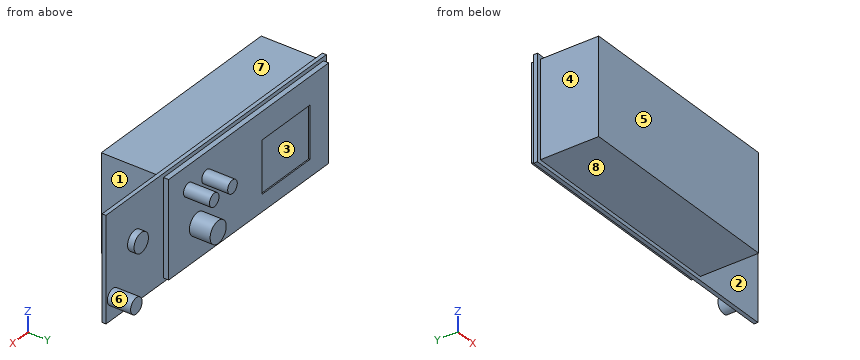
```python
from build123d import *

# Parameters (mm, degrees)
SKETCH_1_W          = 230
SKETCH_1_H          = 80
EXTRUDE_1_DEPTH     = 3
SKETCH_2_W          = 167
SKETCH_2_H          = 74
EXTRUDE_2_DEPTH     = 4
SKETCH_3_W          = 50
SKETCH_3_H          = 40
CUT_EXTRUDE_1_DEPTH = 1
SKETCH_4_R          = 8.4
EXTRUDE_3_DEPTH     = 16
SKETCH_5_R          = 5
EXTRUDE_4_DEPTH     = 20
SKETCH_6_R          = 6
EXTRUDE_5_DEPTH     = 18
SKETCH_7_R          = 7.5
EXTRUDE_6_DEPTH     = 5
SKETCH_8_W          = 167
SKETCH_8_H          = 74
EXTRUDE_7_DEPTH     = 45


with BuildPart() as part:
    # 草图1 → 凸台-拉伸1 (new body)
    with BuildSketch(Plane(origin=(0, 0, 0), x_dir=(1, 0, 0), z_dir=(0, 1, 0))):
        with Locations((35.37586548, -1.78041543)):
            Rectangle(SKETCH_1_W, SKETCH_1_H)
    extrude(amount=EXTRUDE_1_DEPTH)

    # 草图2 → 凸台-拉伸2 (add)
    with BuildSketch(Plane(origin=(0, 3, 0), x_dir=(1, 0, 0), z_dir=(0, 1, 0))):
        with Locations((6.87586548, -1.78041543)):
            Rectangle(SKETCH_2_W, SKETCH_2_H)
    extrude(amount=EXTRUDE_2_DEPTH)

    # 草图3 → 切除-拉伸1 (cut)
    with BuildSketch(Plane(origin=(0, 7, 0), x_dir=(1, 0, 0), z_dir=(0, 1, 0))):
        with Locations((-32.02413452, 2.21958457)):
            Rectangle(SKETCH_3_W, SKETCH_3_H)
    extrude(amount=-CUT_EXTRUDE_1_DEPTH, mode=Mode.SUBTRACT)

    # 草图4 → 凸台-拉伸3 (add)
    with BuildSketch(Plane(origin=(0, 7, 0), x_dir=(1, 0, 0), z_dir=(0, 1, 0))):
        with Locations(Location((60.37586548, 9.21958457, 0), (0, 0, 270))):
            Circle(SKETCH_4_R)
    extrude(amount=EXTRUDE_3_DEPTH)

    # 草图5 → 凸台-拉伸4 (add)
    with BuildSketch(Plane(origin=(0, 7, 0), x_dir=(1, 0, 0), z_dir=(0, 1, 0))):
        with Locations(Location((50.87586548, -20.78041543, 0), (0, 0, 270))):
            Circle(SKETCH_5_R)
        with Locations(Location((69.87586548, -20.78041543, 0), (0, 0, 270))):
            Circle(SKETCH_5_R)
    extrude(amount=EXTRUDE_4_DEPTH)

    # 草图6 → 凸台-拉伸5 (add)
    with BuildSketch(Plane(origin=(0, 3, 0), x_dir=(1, 0, 0), z_dir=(0, 1, 0))):
        with Locations(Location((143.07586548, 21.71958457, 0), (0, 0, 270))):
            Circle(SKETCH_6_R)
    extrude(amount=EXTRUDE_5_DEPTH)

    # 草图7 → 凸台-拉伸6 (add)
    with BuildSketch(Plane(origin=(0, 3, 0), x_dir=(1, 0, 0), z_dir=(0, 1, 0))):
        with Locations(Location((120.37586548, -8.108420441, 0), (0, 0, 270))):
            Circle(SKETCH_7_R)
    extrude(amount=EXTRUDE_6_DEPTH)

    # 草图8 → 凸台-拉伸7 (add)
    with BuildSketch(Plane.XZ):
        with Locations((6.87586548, 1.78041543)):
            Rectangle(SKETCH_8_W, SKETCH_8_H)
    extrude(amount=EXTRUDE_7_DEPTH)


solid = part.part
```
Geometry check sheet. Reference: the model listing, model coordinates, mm. Face numbers are marked on the shaded views. A direction names the side the tool comes from. Give positions to 0.01 mm unless a question says otherwise; leave off trailing zeros. Loops run counter-clockwise (first coordinate to the right, second up) from the corner with the lowest first, then second, coordinate; pieces in that order, holes last. Notation, with made-up numbers: (30.5, 42.25) - (75.5, 42.25) arc R6 cw to (75.5, 49.25) - close; hole circle Ø3 at (46, 41). An arc over 180 degrees is marked (long way). Use CSV: the item, a comma, the result in double quotes. Start each with the question number.
Q1. Scan lines: probe 1 along Y at (x, z) = (9, 23.5); probe 2 along Y at (x, z) = (-51.5, -6); probe 3 along X at (y, z) = (-39.5, 17). Record each from-to range of solid material in increasing order. Write a range as from..to.
Q2. Release check for a two-part mould opening along X. For the marked faces 1, 2, 3 and 4 record: +X half, -X half, draft (parallel to the pull), parting line (faces both ways), or undercut.
Q3. Access from +Z, -Z, +X, -X, +Y, -Y to the whole of each face (thin tool, end or side, straight path). Record for the marked faces 5, 6, 7 and 8.
Q4. Go/stop test with flat-tipped pins: pin 1 Ø22 at (x, z) = (2, 17.5) entering from +Y; pin 2 Ø6 at (x, z) = (145.5, -24.5) entering from +Y; pin 3 Ø13.5 at (x, z) = (56.5, -7.5) entering from +Y. Record where each tip stops, or that it passes through.
Q5. Section check A-A, the plane x = -26. Record the cut outline in (y, z).
Q6. Section check B-B, the plane z = 36. Record the cut outline in (x, y), and give its area (3 significant figures).
Q7. Section check D-D, the plane y = -23. Record the cut outline in (x, z), and give its area (3 significant figures).
Q8. Section check C-C, the plane x = 42. Record the cut outline in (y, z), and give its area (3 significant figures).
Findings below:
1,probe 1,"y = -45..7"
1,probe 2,"y = -45..6"
1,probe 3,"x = -76.62..90.38"
2,face 1,"+X half"
2,face 2,"draft"
2,face 3,"undercut"
2,face 4,"-X half"
3,face 5,"+Z, -Z, +X, -X, -Y"
3,face 6,"+Y"
3,face 7,"+Z, +X, -X, -Y"
3,face 8,"-Z, +X, -X, -Y"
4,pin 1,"stops at y = 7"
4,pin 2,"stops at y = 21"
4,pin 3,"stops at y = 23"
5,outline,"(-45, -35.22) - (0, -35.22) - (0, -38.22) - (3, -38.22) - (3, -35.22) - (7, -35.22) - (7, -22.22) - (6, -22.22) - (6, 17.78) - (7, 17.78) - (7, 38.78) - (3, 38.78) - (3, 41.78) - (0, 41.78) - (0, 38.78) - (-45, 38.78) - close"
6,outline,"(-79.62, 0) - (-76.62, 0) - (-76.62, -45) - (90.38, -45) - (90.38, 0) - (150.38, 0) - (150.38, 3) - (90.38, 3) - (90.38, 7) - (-76.62, 7) - (-76.62, 3) - (-79.62, 3) - close"
6,area,"8,870 mm^2"
7,outline,"(-76.62, -35.22) - (90.38, -35.22) - (90.38, 38.78) - (-76.62, 38.78) - close"
7,area,"12,400 mm^2"
8,outline,"(-45, -35.22) - (0, -35.22) - (0, -38.22) - (3, -38.22) - (3, -35.22) - (7, -35.22) - (7, 38.78) - (3, 38.78) - (3, 41.78) - (0, 41.78) - (0, 38.78) - (-45, 38.78) - close"
8,area,"3,870 mm^2"
